```python
from build123d import *

# Parameters (mm, degrees)
F2_W     = 69.451071322
F2_H     = 59.5968812704
F3_DEPTH = 127
F4_W     = 56.0608096421
F4_H     = 12.9187703133
F5_DEPTH = 55.88
F6_R     = 167.4278885547
F7_DEPTH = 12.7


with BuildPart() as f1:
    # F0 (on Front) → F1 (revolve)
    with BuildSketch(Plane.XZ):
        Polygon((19.2788038403, 161.9556288534), (2.3539757822, 161.9556288534), (2.3539757822, 0), (101.1059731245, 0), (101.1059731245, 81.5908461809), (50.6069213152, 81.5908461809), (50.6069213152, 104.0337234735), (90.3515517712, 104.0337234735), (90.3515517712, 120.3983277082), (44.5283316076, 120.3983277082), (44.5283316076, 140.5034065247), (57.6206743717, 140.5034065247), (57.6206743717, 161.9556288534), align=None)
        Polygon((101.1059731245, 0), (2.3539757822, 0), (2.3539757822, -142.8443711466), (2.3539757822, -161.9556288534), (19.2788038403, -161.9556288534), (57.6206743717, -161.9556288534), (57.6206743717, -140.5034065247), (44.5283316076, -140.5034065247), (44.5283316076, -120.3983277082), (90.3515517712, -120.3983277082), (90.3515517712, -104.0337234735), (50.6069213152, -104.0337234735), (50.6069213152, -81.5908461809), (101.1059731245, -81.5908461809), align=None)
    revolve(axis=Axis((0, 0, 9.5556288534), (0, 0, -1)))

    # F2 (on Front) → F3 (cut, symmetric)
    with BuildSketch(Plane.XZ):
        with Locations((80.894831568, 163.0262359977)):
            Rectangle(F2_W, F2_H)
        with Locations((80.894831568, -163.0262359977)):
            Rectangle(F2_W, F2_H)
    extrude(amount=F3_DEPTH, both=True, mode=Mode.SUBTRACT)

    # F4 (on face) → F5 (join)
    with BuildSketch(Plane.YZ.offset(46.169295907)):
        with Locations((0, 152.1677672863)):
            Rectangle(F4_W, F4_H)
        with Locations((0, -152.1677672863)):
            Rectangle(F4_W, F4_H)
    extrude(amount=F5_DEPTH)

    # F6 (on face) → F7 (join)
    with BuildSketch(Plane.YZ.offset(102.049295907)):
        Circle(F6_R)
    extrude(amount=F7_DEPTH)


solid = f1.part
```
Could you check a few things on this model? Use its own coordinates, in mm. A direction names the side the tool comes from. Coordinates: 2 decimals unless noted, no trailing zeros. Write each loop counter-clockwise with the first axis right and the second up, starting at its lowest first coordinate (ties: lowest second). Pieces come first, ordered by that corner, then holes. Notation, with made-up numbers: (-20.5, 85) -> (25.5, 85) arc R12 cw to (25.5, 107) -> close; hole circle Ø9 at (-20, 51.5). An arc over 180 degrees is marked (long way). Write item = value, one per line. Start each with the question number.
(1) I want a section at A-A (z = 0). Please give me the cut outline in (x, y), plus the area to 4 significant figures.
(2) Will these pins go through, and if not, where does the flat tip stop? pin 1 (8 mm diameter, centred on y = 76, z = -16.5, fed in from -X); pin 2 (6 mm diameter, centred on x = -30.5, y = 37, fed in from +Z); pin 3 (3 mm diameter, centred on x = -50, y = 49, fed in from +Z).
(3) We'd pull the mould along Z, two halves only. Please class faces 6 (the face through (74, 0, -158.627)), 7 (the face through (-46.4, 21.1, 81.591)), 8 (the face through (74, 0, 158.627)): released by +Z, released by -Z, zero draft, split by the parting line, or undercut.
(4) I want a section at B-B (z = 35). Please give me the cut outline in (x, y), plus the area to 3 significant figures.
(5) I need wall thicknesses on line 1 (X direction, y = 0, z = 38); line 2 (X direction, y = 0, z = -82); line 3 (Z direction, x = 79.5, y = -12). Which ranges of each line are inside material? Lowest first, please. Write a range as [from, to].
(6) Which directions (+Z, -Z, +X, -X, +Y, -Y) give clear straight access to the entire face, cutting with the end or side of a thin tool? Please do faces 1 (the face through (74, 28.03, -152)), 2 (the face through (74, -28.03, 152)), 3 (the face through (46.169, 0, 144)), 4 (the face through (-5, -1, -161.956)), 5 (the face through (74, 0, 145.708)).
Result set:
q1.outline = circle Ø202.21 at (0, 0); (102.05, -167.43) -> (114.75, -167.43) -> (114.75, 167.43) -> (102.05, 167.43) -> close; hole circle Ø4.71 at (0, 0)
q1.area = 36,350 mm2
q2.pin_1 = -70.98
q2.pin_2 = 161.96
q2.pin_3 = 120.4
q3.face_6 = released by -Z
q3.face_7 = undercut
q3.face_8 = released by +Z
q4.outline = circle Ø202.21 at (0, 0); (102.05, -163.73) -> (114.75, -163.73) -> (114.75, 163.73) -> (102.05, 163.73) -> close; hole circle Ø4.71 at (0, 0)
q4.area = 36,300 mm2
q5.line_1 = [-101.11, -2.35], [2.35, 101.11], [102.05, 114.75]
q5.line_2 = [-50.61, -2.35], [2.35, 50.61], [102.05, 114.75]
q5.line_3 = [-158.63, -145.71], [-120.4, -104.03], [-81.59, 81.59], [104.03, 120.4], [145.71, 158.63]
q6.face_1 = -Z, +Y
q6.face_2 = +Z, -Y
q6.face_3 = none
q6.face_4 = -Z, -X, +Y, -Y
q6.face_5 = +Y, -Y
